Design review of the part built by this model. Coordinates are the model's own, in mm. A direction names the side the tool comes from. Give positions to 0.01 mm unless a question says otherwise; leave off trailing zeros. Write each loop counter-clockwise with the first axis right and the second up, starting at its lowest first coordinate (ties: lowest second). Pieces come first, ordered by that corner, then holes. Notation, with made-up numbers: (48.5, 64.5) -> (99.5, 64.5) arc R28 ccw to (99.5, 95.5) -> close; hole circle Ø8 at (11, 47.25). An arc over 180 degrees is marked (long way). Answer as a JSON object with one key per item and string values.
```python
from build123d import *

# Parameters (mm, degrees)
BOSS_EXTRUDE1_DEPTH     = 10
BOSS_EXTRUDE2_DEPTH     = 3
CUT_EXTRUDE1_DEPTH      = 39.52596527
CUT_EXTRUDE1_DEPTH_BACK = 39.52596527
CUT_EXTRUDE2_DEPTH      = 39.52596527


with BuildPart() as part:
    # Sketch1 → Boss-Extrude1 (new, symmetric)
    with BuildSketch(Plane.XY):
        Polygon((0, 0), (0, 28), (3.5, 28), (3.5, 3.5), (28, 3.5), (28, 0), align=None)
    extrude(amount=BOSS_EXTRUDE1_DEPTH, both=True)

    # Sketch2 → Boss-Extrude2 (add)
    with BuildSketch(Plane.XY.offset(10)):
        Polygon((28, 5.5), (28, 3.5), (3.5, 3.5), (3.5, 28), (5.5, 28), (5.5, 23), (23, 5.5), align=None)
    boss_extrude2 = extrude(amount=-BOSS_EXTRUDE2_DEPTH)

    # Mirror1: Boss-Extrude2 across plane
    add(boss_extrude2.mirror(Plane.XY))

    # Sketch3 → Cut-Extrude1 (cut, two sides: drawn at the far end of the back side and taken through both)
    with BuildSketch(Plane(origin=(0, 3.5, 0), x_dir=(1, 0, 0), z_dir=(0, 1, 0)).offset(-CUT_EXTRUDE1_DEPTH_BACK)):
        with BuildLine():
            ThreePointArc((19, 0), (16.584170789, 3.141123858), (12.928209788, 1.61245155))
            Line((12.928209788, 1.61245155), (18.571790212, -1.61245155))
            ThreePointArc((18.571790212, -1.61245155), (18.891123858, -0.834170789), (19, 0))
        make_face()
        with BuildLine():
            Line((18.571790212, -1.61245155), (12.928209788, 1.61245155))
            ThreePointArc((12.928209788, 1.61245155), (14.13754845, -2.821790212), (18.571790212, -1.61245155))
        make_face()
    extrude(amount=CUT_EXTRUDE1_DEPTH + CUT_EXTRUDE1_DEPTH_BACK, mode=Mode.SUBTRACT)

    # Sketch4 → Cut-Extrude2 (cut, through all)
    with BuildSketch(Plane(origin=(3.5, 0, 0), x_dir=(0, 0, -1), z_dir=(1, 0, 0))):
        with BuildLine():
            ThreePointArc((3.25, 15.75), (2.810957803, 17.381262159), (1.61245155, 18.571790212))
            Line((1.61245155, 18.571790212), (-1.61245155, 12.928209788))
            ThreePointArc((-1.61245155, 12.928209788), (1.631262159, 12.939042197), (3.25, 15.75))
        make_face()
        with BuildLine():
            Line((-1.61245155, 12.928209788), (1.61245155, 18.571790212))
            ThreePointArc((1.61245155, 18.571790212), (-2.821790212, 17.36245155), (-1.61245155, 12.928209788))
        make_face()
    extrude(amount=-CUT_EXTRUDE2_DEPTH, mode=Mode.SUBTRACT)


solid = part.part
```
(1) For line 1 along Z through (x, y) = (8, 18.75); line 2 along Y through (x, z) = (26.25, 0.5), list the stretches that pass through material, from the lowest coordinate up.
Here are the results:
{"line 1": "z = -10 to -7, 7 to 10", "line 2": "y = 0 to 3.5"}
(2) For faces 1 (the flat face through (10, 10, 7)), 2 (the flat face through (0, 11, 0)), 3 (the flat face through (5.5, 26, -9)), list the 3-axis set-ups (+Z, -Z, +X, -X, +Y, -Y) from which the entire face can be reached by the end or side of a thin tool; tool diameter is ignored.
Here are the results:
{"face 1": "+X, +Y", "face 2": "+Z, -Z, -X, +Y, -Y", "face 3": "+Z, -Z, +X, +Y"}
(3) We need section B-B, the plane x = 15.75. State the section outline as (y, z) points, then the cut area to 3 significant figures.
Here are the results:
{"outline": "(0, -10) -> (12.75, -10) -> (12.75, -7) -> (3.5, -7) -> (3.5, -3.25) -> (0, -3.25) -> close; (0, 3.25) -> (3.5, 3.25) -> (3.5, 7) -> (12.75, 7) -> (12.75, 10) -> (0, 10) -> close", "area": "103 mm²"}
(4) We need section C-C, the plane z = 1. State the section outline as (x, y) points.
Here are the results:
{"outline": "(0, 0) -> (12.66, 0) -> (12.66, 3.5) -> (3.5, 3.5) -> (3.5, 12.66) -> (0, 12.66) -> close; (0, 18.84) -> (3.5, 18.84) -> (3.5, 28) -> (0, 28) -> close; (18.84, 0) -> (28, 0) -> (28, 3.5) -> (18.84, 3.5) -> close"}
(5) We need section A-A, the plane y = 14.5. State the section outline as (x, z) points, then the cut area to 3 significant figures.
Here are the results:
{"outline": "(0, -10) -> (14, -10) -> (14, -7) -> (3.5, -7) -> (3.5, -3) -> (0, -3) -> close; (0, 3) -> (3.5, 3) -> (3.5, 7) -> (14, 7) -> (14, 10) -> (0, 10) -> close", "area": "112 mm²"}
(6) Clearance check with flat-ended pins moving along their axes: pin 1 (2.5 mm diameter, centred on x = 26.5, z = 9, fed in from +Y); pin 2 (4 mm diameter, centred on x = 20.5, z = 1, fed in from +Y); pin 3 (12 mm diameter, centred on y = 11.5, z = 6.5, fed in from -X); pin 4 (0.9 mm diameter, centred on y = 25, z = 9, fed in from +X). State where each tip first meets the part, or that it passes through.
Here are the results:
{"pin 1": "stops at y = 5.5", "pin 2": "stops at y = 3.5", "pin 3": "stops at x = 0", "pin 4": "stops at x = 5.5"}
(7) We need section D-D, the plane y = 26. State the section outline as (x, z) points, then the cut area to 3 significant figures.
Here are the results:
{"outline": "(0, -10) -> (5.5, -10) -> (5.5, -7) -> (3.5, -7) -> (3.5, 7) -> (5.5, 7) -> (5.5, 10) -> (0, 10) -> close", "area": "82.0 mm²"}
